Could you check a few things on this drawing? It's one solid part, dimensions in mm from its lowest x, y, z. A direction names the side the tool comes from. Give positions to 0.01 mm unless a question says otherwise; leave off trailing zeros. Order: outer loops, then holes, each group sorted by start corner. A loop starts at its lowest first (then second) coordinate and runs counter-clockwise, first axis right, second up. Notation, with made-up numbers: (38, 85.25) -> (60, 85.25) arc R16 ccw to (60, 101.25) -> close; hole circle Ø7 at (65, -6.75). An arc over 180 degrees is marked (long way). Write each question's results on one line, items separated by ' | '. Start each with the question number.
Q1. Imagine slicing it at A-A, the plane z = 5.5. Please give me the cut outline in (x, y).
Q2. Imagine slicing it at B-B, the plane x = 7.25. Please give me the cut outline in (y, z) (1 decimal).
Q3. For the marked faces 1 and 2, which set-ups out of +Z, -Z, +X, -X, +Y, -Y let a thin tool reach every point of the face, with its end or its side?
Q4. Imagine slicing it at D-D, the plane y = 3.05. Please give me the cut outline in (x, z) (1 decimal).
Q5. I'm going to push a flat-ended pin straight in: pin 1 (2 mm diameter, centred on x = 4, z = 4, fed in from +Y). Where does the tip first touch, or does it pass through?
Q6. Thinking about a two-plate mould opening in Z: for the marked faces 3, 4 and 5, which applies, pulls with the +Z half, pulls with the -Z half, needs draft (parallel to the pull), parting line crosses it, or undercut?
Q7. I need wall thicknesses on line 1 along X through (y, z) = (1.7, 3.5); line 2 along Z through (x, y) = (5, 0.25); line 3 along Z through (x, y) = (6.5, 2.15) (1 decimal). Which ranges of each line are inside material? Lowest first, please. Write a range as [from, to].
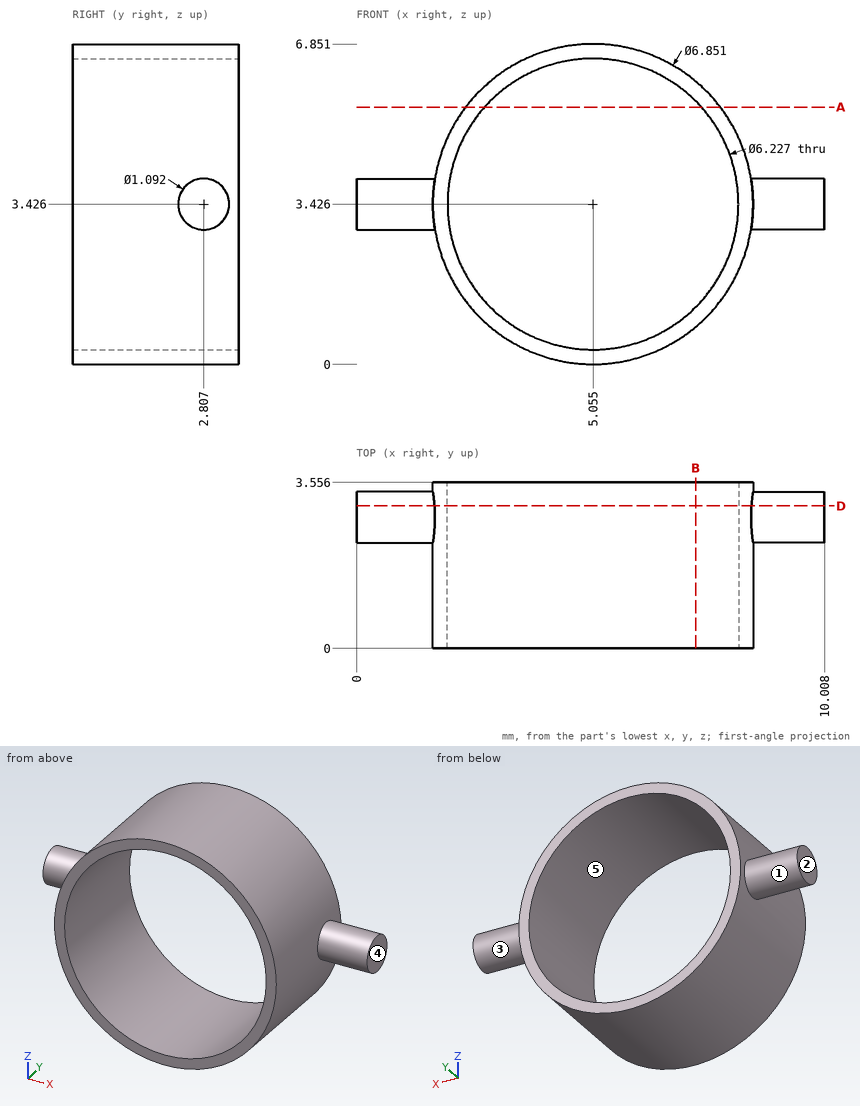
Geometry check:
1) outline: (2.33, 0) -> (2.73, 0) -> (2.73, 3.56) -> (2.33, 3.56) -> close; (7.38, 0) -> (7.78, 0) -> (7.78, 3.56) -> (7.38, 3.56) -> close
2) outline: (0, 0.8) -> (3.6, 0.8) -> (3.6, 1.2) -> (0, 1.2) -> close; (0, 5.6) -> (3.6, 5.6) -> (3.6, 6.1) -> (0, 6.1) -> close
3) face 1: -X | face 2: +Z, -Z, -X, +Y, -Y
4) outline: (0, 2.9) -> (1.7, 2.9) arc R3.4 ccw to (8.4, 2.9) -> (10, 2.9) -> (10, 3.9) -> (8.4, 3.9) arc R3.4 ccw to (1.7, 3.9) -> (0, 3.9) -> close; hole circle Ø6.2 at (5.1, 3.4)
5) pin 1: through
6) face 3: parting line crosses it | face 4: needs draft | face 5: undercut
7) line 1: [1.63, 1.94], [8.17, 8.48] | line 2: [0, 0.31], [6.54, 6.85] | line 3: [0.3, 0.7], [6.2, 6.5]
